from build123d import *

# Parameters (mm, degrees)
CROQUIS1_W              = 98
CROQUIS1_H              = 60
SALIENTE_EXTRUIR1_DEPTH = 0.8
CROQUIS2_R              = 1.5
CORTAR_EXTRUIR1_DEPTH   = 2.6
CROQUIS3_W              = 97
CROQUIS3_H              = 40
SALIENTE_EXTRUIR2_DEPTH = 9.5
CROQUIS4_W              = 76
CROQUIS4_H              = 25.2
CORTAR_EXTRUIR2_DEPTH   = 1
CORTAR_EXTRUIR5_START   = -8.5
CROQUIS5_R              = 0.5
CORTAR_EXTRUIR5_DEPTH   = 0.001
CROQUIS5_2_R            = 0.5
CORTAR_EXTRUIR6_DEPTH   = 11.1
MATRIZL1_COUNT          = 16
MATRIZL1_PITCH          = 2.54


with BuildPart() as part:
    # Croquis1 → Saliente-Extruir1 (new body, symmetric)
    with BuildSketch(Plane.XY):
        Rectangle(CROQUIS1_W, CROQUIS1_H)
    extrude(amount=SALIENTE_EXTRUIR1_DEPTH, both=True)

    # Croquis2 → Cortar-Extruir1 (cut, through all)
    with BuildSketch(Plane.XY.offset(0.8)):
        with Locations((-46.5, 27.5)):
            Circle(CROQUIS2_R)
        with Locations((-46.5, -27.5)):
            Circle(CROQUIS2_R)
        with Locations((46.5, -27.5)):
            Circle(CROQUIS2_R)
        with Locations((46.5, 27.5)):
            Circle(CROQUIS2_R)
    extrude(amount=-CORTAR_EXTRUIR1_DEPTH, mode=Mode.SUBTRACT)

    # Croquis3 → Saliente-Extruir2 (add)
    with BuildSketch(Plane.XY.offset(0.8)):
        Rectangle(CROQUIS3_W, CROQUIS3_H)
    extrude(amount=SALIENTE_EXTRUIR2_DEPTH)

    # Croquis4 → Cortar-Extruir2 (cut)
    with BuildSketch(Plane.XY.offset(10.3)):
        Rectangle(CROQUIS4_W, CROQUIS4_H)
    extrude(amount=-CORTAR_EXTRUIR2_DEPTH, mode=Mode.SUBTRACT)

    # Croquis5 → Cortar-Extruir5 (cut)
    with BuildSketch(Plane.XY.offset(9.3).offset(CORTAR_EXTRUIR5_START)):
        with BuildLine():
            Line((-39.9, 30), (-38.1, 30))
            Line((-38.1, 30), (-38.1, 27.5))
            ThreePointArc((-38.1, 27.5), (-39, 26.6), (-39.9, 27.5))
            Line((-39.9, 27.5), (-39.9, 30))
        make_face()
        with Locations((-39, 27.5)):
            Circle(CROQUIS5_R, mode=Mode.SUBTRACT)
    cortar_extruir5 = extrude(amount=-CORTAR_EXTRUIR5_DEPTH, mode=Mode.SUBTRACT)

    # Croquis5<2> → Cortar-Extruir6 (cut, through all)
    with BuildSketch(Plane.XY.offset(9.3)):
        with Locations((-39, 27.5)):
            Circle(CROQUIS5_2_R)
    cortar_extruir6 = extrude(amount=-CORTAR_EXTRUIR6_DEPTH, mode=Mode.SUBTRACT)

    # MatrizL1: Cortar-Extruir5, Cortar-Extruir6 ×16
    with Locations(*[(i * MATRIZL1_PITCH, 0, 0) for i in range(1, MATRIZL1_COUNT)]):
        add(cortar_extruir5, mode=Mode.SUBTRACT)
        add(cortar_extruir6, mode=Mode.SUBTRACT)


solid = part.part
The listing builds one solid part. Answer for the finished solid, in the listing's coordinates (mm). A direction names the side the tool comes from. Give positions to 0.01 mm unless a question says otherwise; leave off trailing zeros. Loops run counter-clockwise (first coordinate to the right, second up) from the corner with the lowest first, then second, coordinate; pieces in that order, holes last. Notation, with made-up numbers: (84, 19) - (97, 19) arc R17 ccw to (97, 46) - close; hole circle Ø10 at (11, -6). An arc over 180 degrees is marked (long way). Answer as a JSON object with one key per item and string values.
1. A cutting plane is placed at C-C (x = 22). Write down the section's boundary in (y, z).
Determined:
{"outline": "(-30, -0.8) - (30, -0.8) - (30, 0.8) - (20, 0.8) - (20, 10.3) - (12.6, 10.3) - (12.6, 9.3) - (-12.6, 9.3) - (-12.6, 10.3) - (-20, 10.3) - (-20, 0.8) - (-30, 0.8) - close"}
2. Flat-ended cylindrical pins translate along their axes: pin 1 Ø1.4 at (x, y) = (-8, 27.5) entering from +Z; pin 2 Ø2 at (x, y) = (31.5, -5.5) entering from +Z; pin 3 Ø3 at (y, z) = (4.5, 7.5) entering from -X. Find the tip coordinate at first contact, or state that the pin passes through.
Determined:
{"pin 1": "z = 0.8", "pin 2": "z = 9.3", "pin 3": "x = -48.5"}
3. A cutting plane is placed at A-A (y = -27.5). Write down the section's boundary in (x, z), then the cut area to 3 significant figures.
Determined:
{"outline": "(-49, -0.8) - (-48, -0.8) - (-48, 0.8) - (-49, 0.8) - close; (-45, -0.8) - (45, -0.8) - (45, 0.8) - (-45, 0.8) - close; (48, -0.8) - (49, -0.8) - (49, 0.8) - (48, 0.8) - close", "area": "147 mm²"}
4. A cutting plane is placed at D-D (y = 6.5). Write down the section's boundary in (x, z), then the cut area to 3 significant figures.
Determined:
{"outline": "(-49, -0.8) - (49, -0.8) - (49, 0.8) - (48.5, 0.8) - (48.5, 10.3) - (38, 10.3) - (38, 9.3) - (-38, 9.3) - (-38, 10.3) - (-48.5, 10.3) - (-48.5, 0.8) - (-49, 0.8) - close", "area": "1,000 mm²"}
5. For a pull along X with two mould halves and no side action, classify faces 4 (the flat face through (-16, 29, 0.799)), 5 (the flat face through (-48.5, 0, 5)), 6 (the flat face through (48.5, 0, 5)), 7 (the cylindrical face through (45.39, -26.49, 0.01)) as pulls with the +X half, pulls with the -X half, needs draft (parallel to the pull), parting line crosses it, or undercut.
Determined:
{"face 4": "needs draft", "face 5": "pulls with the -X half", "face 6": "pulls with the +X half", "face 7": "undercut"}
6. A cutting plane is placed at B-B (x = 46.5). Write down the section's boundary in (y, z).
Determined:
{"outline": "(-30, -0.8) - (-29, -0.8) - (-29, 0.8) - (-30, 0.8) - close; (-26, -0.8) - (26, -0.8) - (26, 0.8) - (20, 0.8) - (20, 10.3) - (-20, 10.3) - (-20, 0.8) - (-26, 0.8) - close; (29, -0.8) - (30, -0.8) - (30, 0.8) - (29, 0.8) - close"}
7. Find the intervals of material crossed by L1, parallel to Y at x = -46.5, z = -0.05; L2, parallel to Y at x = -0.9, z = 0.1; L3, parallel to X at y = -17, z = 4.25, in increasing order. Write a range as [from, to].
Determined:
{"L1": "[-30, -29], [-26, 26], [29, 30]", "L2": "[-30, 27], [28, 30]", "L3": "[-48.5, 48.5]"}
8. For faces 1 (the flat face through (-26, 29, 0.799)), 2 (the flat face through (-1, 0, 9.3)), 3 (the cylindrical face through (-47.61, 28.51, 0.01)), determine the directions among +Z, -Z, +X, -X, +Y, -Y from which every point of the face is accessible in a straight line to the end or side of a thin tool.
Determined:
{"face 1": "+Z, +X, -X, +Y", "face 2": "+Z", "face 3": "+Z, -Z"}
